Autodesk Inventor part; units mm, degrees
ref_plane "YZ Plane" through (0, 0, 0) normal (1, 0, 0) x (0, 1, 0)
ref_plane "XZ Plane" through (0, 0, 0) normal (0, 1, 0) x (-1, 0, 0)
ref_plane "XY Plane" through (0, 0, 0) normal (0, 0, 1) x (1, 0, 0)
sketch "スケッチ1" plane through (0, 0, 0) normal (0, 0, 1) x (1, 0, 0)
  line L0 (-4, 4) -> (4, 4)
  line L1 (4, 4) -> (4, 2.15)
  line L2 (4, 2.15) -> (-4, 2.15)
  line L3 (-4, 2.15) -> (-4, 4)
  line L4 (0, 0) -> (0, 4.5155) construction
  line L5 (0, 0) -> (8.3877, 0) construction
  dimension "d0" = 8
  dimension "d1" = 4.3
  dimension "d2" = 8
revolve "回転1" add sketch "スケッチ1" angle 360 about axis through (0, 0, 0) along (1, 0, 0)
chamfer "面取り1" distance 0.3 angle 45 2 edges at (4, -4, 0) (-4, -4, 0)
sketch "スケッチ2" plane through (4, 0, 0) normal (1, 0, 0) x (0, 0, -1)
  point P0 (0, 0)
  point P1 (0, 0)
hole "穴1" at (4, 0, 0) direction (-1, 0, 0) diameter 6 depth 2.5 tip angle 118 counterbore diameter 7.3 counterbore depth 0.65
mirror "ミラー1" about plane through (0, 0, 0) normal (1, 0, 0) of "穴1"
properties part number "BELT_SUPPORT_OUTER"
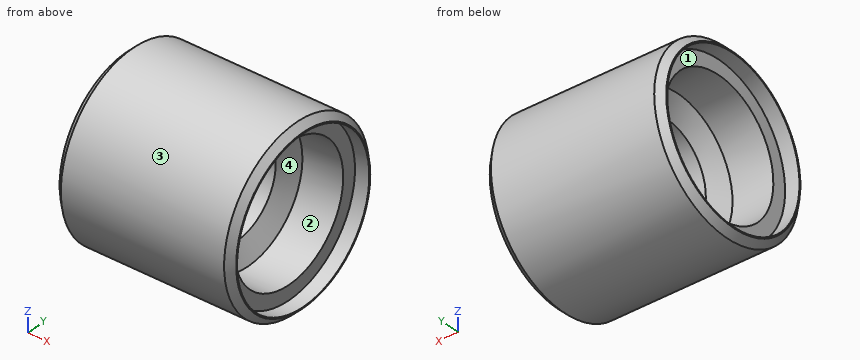
Input: part model. Units: mm. Frame: model coordinates. Face numbers are marked on the shaded views. A direction names the side the tool comes from. Coordinates: 2 decimals unless noted, no trailing zeros. Loops run counter-clockwise (first coordinate to the right, second up) from the corner with the lowest first, then second, coordinate; pieces in that order, holes last. Notation, with made-up numbers: (46.5, -31) -> (50.5, -31) arc R20 ccw to (50.5, -8) -> close; hole circle Ø9 at (-33.5, 52). An arc over 180 degrees is marked (long way). Use a Markdown table: item, result.
1) Pull-direction query (Z, two-part tool) for the marked faces 3 and 4; classes: released by +Z, released by -Z, zero draft, split by the parting line, or undercut.
Results found:
| item | result |
|---|---|
| face 3 | split by the parting line |
| face 4 | undercut |
2) Cut plane A-A (z = 0). Return the cut outline in (x, y), then the cut area to 3 significant figures.
Results found:
| item | result |
|---|---|
| outline | (-4, -3.7) -> (-3.7, -4) -> (3.7, -4) -> (4, -3.7) -> (4, -3.65) -> (3.35, -3.65) -> (3.35, -3) -> (1.5, -3) -> (0.99, -2.15) -> (-0.99, -2.15) -> (-1.5, -3) -> (-3.35, -3) -> (-3.35, -3.65) -> (-4, -3.65) -> close; (-4, 3.65) -> (-3.35, 3.65) -> (-3.35, 3) -> (-1.5, 3) -> (-0.99, 2.15) -> (0.99, 2.15) -> (1.5, 3) -> (3.35, 3) -> (3.35, 3.65) -> (4, 3.65) -> (4, 3.7) -> (3.7, 4) -> (-3.7, 4) -> (-4, 3.7) -> close |
| area | 18.4 mm2 |
3) Cut plane D-D (x = 0.25). Return the cut outline in (y, z), then the cut area to 3 significant figures.
Results found:
| item | result |
|---|---|
| outline | circle Ø8 at (0, 0); hole circle Ø4.3 at (0, 0) |
| area | 35.7 mm2 |
4) Cut plane C-C (x = -2.75). Return the cut outline in (y, z).
Results found:
| item | result |
|---|---|
| outline | circle Ø8 at (0, 0); hole circle Ø6 at (0, 0) |
5) Material intervals for line 1 along Z through (x, y) = (2.65, 0); line 2 along X through (y, z) = (2.5, -2.5); line 3 along Y through (x, z) = (2, -1.75), sorted ascending. Write a range as from..to.
Results found:
| item | result |
|---|---|
| line 1 | z = -4..-3, 3..4 |
| line 2 | x = -3.35..3.35 |
| line 3 | y = -3.6..-2.44, 2.44..3.6 |
6) Access query for the marked faces 1 and 2. Directions: +Z, -Z, +X, -X, +Y, -Y. A direction counts if a zero-diameter tool reaches every point of the face in a straight line with its end or side. Return the directions, or none.
Results found:
| item | result |
|---|---|
| face 1 | -X |
| face 2 | +X |
7) Contact query for flat-ended pins moving along their axis: pin 1 (1 mm diameter, centred on x = 1, z = -3, fed in from -Y); pin 2 (2 mm diameter, centred on y = -1.5, z = 0.5, fed in from -X); pin 3 (1 mm diameter, centred on x = -2.5, y = -2.5, fed in from -Z). Output: stop coordinate, or through.
Results found:
| item | result |
|---|---|
| pin 1 | stops at y = -3.12 |
| pin 2 | stops at x = -1.25 |
| pin 3 | stops at z = -3.46 |
